```python
from build123d import *

# Parameters (mm, degrees)
SKETCH_1_W      = 85
SKETCH_1_H      = 54
SKETCH_1_R      = 1.5
EXTRUDE_1_DEPTH = 2
FILLET_1_R      = 5


with BuildPart() as part:
    # 草图1 → 凸台-拉伸1 (new body)
    with BuildSketch(Plane.XY):
        Rectangle(SKETCH_1_W, SKETCH_1_H)
        with Locations((39.5, 0)):
            Circle(SKETCH_1_R, mode=Mode.SUBTRACT)
        with Locations((35.3, 0)):
            Circle(SKETCH_1_R, mode=Mode.SUBTRACT)
        with Locations((0, 14.5)):
            Circle(SKETCH_1_R, mode=Mode.SUBTRACT)
        with Locations((-16, 0)):
            Circle(SKETCH_1_R, mode=Mode.SUBTRACT)
        with Locations((16, 0)):
            Circle(SKETCH_1_R, mode=Mode.SUBTRACT)
        with Locations((0, -14.5)):
            Circle(SKETCH_1_R, mode=Mode.SUBTRACT)
    extrude(amount=EXTRUDE_1_DEPTH)

    # 圆角1
    fillet_1_edges = [part.edges().sort_by_distance(p)[0] for p in [
        (42.5, -27, 1),
        (-42.5, -27, 1),
        (-42.5, 27, 1),
        (42.5, 27, 1),
    ]]
    fillet(fillet_1_edges, radius=FILLET_1_R)


solid = part.part
```
Here's how the part is built. I have some questions about the finished solid (model axes, mm). Coordinates: 2 decimals unless noted, no trailing zeros. Order: outer loops, then holes, each group sorted by start corner. A loop starts at its lowest first (then second) coordinate and runs counter-clockwise, first axis right, second up.
1) Imagine slicing it at A-A on y = -14.5. List the corners of the cut face in (x, z) for me, and give its area (3 significant figures).
2) Will this pin go through, and if not, where does the flat tip stop? pin 1 (4 mm diameter, centred on x = 16, y = 0, fed in from -Z).
3) I need wall thicknesses on line 1 (Y direction, x = 0, z = 0.85); line 2 (Y direction, x = 16, z = 0.8); line 3 (X direction, y = 1, z = 0.4). Which ranges of each line are inside material? Lowest first, please.
4) Imagine slicing it at B-B on x = 16. List the corners of the cut face in (y, z) for me, and give its area (3 significant figures).
5) We'd pull the mould along X, two halves only. Please class faces 1 (the face through (14.5, 0.07, 0.99)), 2 (the face through (41, -25.57, 1.01)), 3 (the face through (-41.07, -25.5, 1.01)): +X half, -X half, draft (parallel to the pull), parting line (faces both ways), or undercut.
Response values:
1. outline: (-42.5, 0) - (-1.5, 0) - (-1.5, 2) - (-42.5, 2) - close; (1.5, 0) - (42.5, 0) - (42.5, 2) - (1.5, 2) - close
1. area: 164 mm2
2. pin 1: stops at z = 0
3. line 1: y = -27 to -16, -13 to 13, 16 to 27
3. line 2: y = -27 to -1.5, 1.5 to 27
3. line 3: x = -42.5 to -17.12, -14.88 to 14.88, 17.12 to 34.18, 36.42 to 38.38, 40.62 to 42.5
4. outline: (-27, 0) - (-1.5, 0) - (-1.5, 2) - (-27, 2) - close; (1.5, 0) - (27, 0) - (27, 2) - (1.5, 2) - close
4. area: 102 mm2
5. face 1: undercut
5. face 2: +X half
5. face 3: -X half
